The listing builds one solid part. Answer for the finished solid, in the listing's coordinates (mm). A direction names the side the tool comes from. Round coordinates to 2 decimals unless told otherwise and drop trailing zeros. Write each loop counter-clockwise with the first axis right and the second up, starting at its lowest first coordinate (ties: lowest second). Pieces come first, ordered by that corner, then holes. Notation, with made-up numbers: M -17.75,21.5 L 38.25,21.5 A17 cw 38.25,31.5 Z; hole C -0.75,87.25 d3. An arc over 180 degrees is marked long. Answer as CSV lines item,"result". Start each with the question number.
Autodesk Inventor part; units mm, degrees
ref_plane "YZ Plane" through (0, 0, 0) normal (1, 0, 0) x (0, 1, 0)
ref_plane "XZ Plane" through (0, 0, 0) normal (0, 1, 0) x (-1, 0, 0)
ref_plane "XY Plane" through (0, 0, 0) normal (0, 0, 1) x (1, 0, 0)
sketch "Skizze4" plane through (0, 0, 0) normal (0, 0, 1) x (1, 0, 0)
  line L0 (0, 0) -> (0, 2)
  line L1 (0, 2) -> (22, 2)
  line L2 (22, 2) -> (22, -6)
  line L3 (22, -6) -> (37, -6)
  line L4 (37, -6) -> (37, 74)
  line L5 (37, 74) -> (61, 74)
  line L6 (61, 74) -> (61, -8)
  line L7 (61, 74) -> (143, 74) construction
  line L8 (61, -8) -> (20, -8)
  line L9 (20, -8) -> (20, 0)
  line L10 (20, 0) -> (0, 0)
  dimension "d2" = 2
  dimension "d3" = 22
  dimension "d4" = 8
  dimension "d5" = 15
  dimension "d6" = 80
  dimension "d7" = 24
  dimension "d8" = 82
  dimension "d9" = 90
  dimension "d10" = 41
extrude "Extrusion3" add sketch "Skizze4" against normal blind 24
sketch "Skizze8" plane through (37, 74, 0) normal (0, 1, 0) x (1, 0, 0)
  line L0 (2, 2) -> (22, 2)
  line L1 (22, 2) -> (22, 22)
  line L2 (22, 22) -> (2, 22)
  line L3 (2, 22) -> (2, 2)
  point P0 (-37, 0)
  dimension "d23" = 20
  dimension "d24" = 20
extrude "Extrusion5" cut sketch "Skizze8" against normal blind 200
sketch "Sketch9" plane through (0, 2, 0) normal (0, 1, 0) x (1, 0, 0)
  point P0 (0, 0)
properties part number "flexibler_standfuß_v0.3"
Q1. For faces 1 (the face through (10, 0, -12)), 2 (the face through (29, -6, -12)), 3 (the face through (59, 34, -12)), determine the directions among +Z, -Z, +X, -X, +Y, -Y from which every point of the face is accessible in a straight line to the end or side of a thin tool.
Q2. Find section A-A (y = 1). Determine the outline of the cut face in (x, z).
Q3. Find section D-D (x = 31). Determine the outline of the cut face in (y, z), plus the area to 3 significant figures.
Q4. Straight lines are drawn through the part: L1, parallel to Z at x = 54, y = 33; L2, parallel to X at y = 11, z = -14.5; L3, parallel to X at y = 57.5, z = -23. For each, find the intervals that lie inside material, in ascending order.
Q5. The mould has two halves that part along X. Classify faces 4 (the face through (61, 34, -12)), 5 (the face through (11, 2, -12)), 6 (the face through (39, 34, -12)): +X half, -X half, draft (parallel to the pull), parting line (faces both ways), or undercut.
Q6. Find section B-B (z = -17). Determine the outline of the cut face in (x, y), plus the area to 3 significant figures.
Q7. Each of these flat-tipped pins is pushed along its axis until it touches: P1, Ø12, axis at y = 43, z = -11, coming from the -X side; P2, Ø12, axis at x = 27, z = -10.5, coming from the +Y side; P3, Ø16, axis at x = 51, y = 45.5, coming from the +Z side; P4, Ø1.5, axis at x = 41.5, z = -3.5, coming from the -Y side. Where does it stop, or does it pass through?
Q8. Find section C-C (y = 17). Determine the outline of the cut face in (x, z), plus the area to 3 significant figures.
Reported:
1,face 1,"+Z, -Z, -X, -Y"
1,face 2,"+Z, -Z, +Y"
1,face 3,"+Y, -Y"
2,outline,"M 0,-24 L 22,-24 L 22,0 L 0,0 Z; M 37,-24 L 61,-24 L 61,0 L 37,0 Z; hole M 39,-22 L 59,-22 L 59,-2 L 39,-2 Z"
3,outline,"M -8,-24 L -6,-24 L -6,0 L -8,0 Z"
3,area,"48.0 mm2"
4,L1,"z = -24 to -22, -2 to 0"
4,L2,"x = 37 to 39, 59 to 61"
4,L3,"x = 37 to 61"
5,face 4,"+X half"
5,face 5,"draft"
5,face 6,"undercut"
6,outline,"M 0,0 L 20,0 L 20,-8 L 39,-8 L 39,74 L 37,74 L 37,-6 L 22,-6 L 22,2 L 0,2 Z; M 59,-8 L 61,-8 L 61,74 L 59,74 Z"
6,area,"418 mm2"
7,P1,"stops at x = 37"
7,P2,"stops at y = 2"
7,P3,"stops at z = 0"
7,P4,"passes through"
8,outline,"M 37,-24 L 61,-24 L 61,0 L 37,0 Z; hole M 39,-22 L 59,-22 L 59,-2 L 39,-2 Z"
8,area,"176 mm2"
